Design review of the part built by this model. Coordinates are the model's own, in mm. A direction names the side the tool comes from. Give positions to 0.01 mm unless a question says otherwise; leave off trailing zeros. Order: outer loops, then holes, each group sorted by start corner. A loop starts at its lowest first (then second) coordinate and runs counter-clockwise, first axis right, second up. Notation, with made-up numbers: (-2.5, -9.75) -> (19.5, -9.75) arc R28 ccw to (19.5, 15.25) -> close; hole circle Ø4 at (-9.75, -7.5). An arc over 180 degrees is marked (long way). Answer in a Markdown table with one row per item. Add a question column.
```python
from build123d import *

# Parameters (mm, degrees)
F0_R     = 4.0005
F0_R_2   = 2.9972
F1_DEPTH = 2.032
F2_R     = 2.54
F3_DEPTH = 5.08
F4_R     = 1.9939
F5_DEPTH = 7.2898
F6_R     = 1.781887
F7_DEPTH = 0.254


with BuildPart() as f1:
    # F0 (on Front) → F1 (new body)
    with BuildSketch(Plane.XZ):
        Circle(F0_R)
        Circle(F0_R_2, mode=Mode.SUBTRACT)
        Circle(F0_R_2)
    extrude(amount=F1_DEPTH)

    # F2 (on face) → F3 (join)
    with BuildSketch(Plane(origin=(0, 0, 0), x_dir=(-1, 0, 0), z_dir=(0, 1, 0))):
        Circle(F2_R)
    extrude(amount=F3_DEPTH)

    # F4 (on face) → F5 (join)
    with BuildSketch(Plane(origin=(0, 5.08, 0), x_dir=(-1, 0, 0), z_dir=(0, 1, 0))):
        Circle(F4_R)
    extrude(amount=F5_DEPTH)

    # F6 (on face) → F7 (join)
    with BuildSketch(Plane(origin=(0, 12.3698, 0), x_dir=(-1, 0, 0), z_dir=(0, 1, 0))):
        Circle(F6_R)
    extrude(amount=F7_DEPTH)


solid = f1.part
```
1) Clearance check with flat-ended pins moving along their axes: P1, Ø2, axis at x = 2.5, y = 9, coming from the -Z side; P2, Ø4, axis at y = 2.5, z = -1, coming from the +X side; P3, Ø4, axis at y = 6.5, z = -2.5, coming from the -X side. State where each tip first meets the part, or that it passes through.
2) Machinability: for faces 1 (the face through (-0.9, -1, -3.9)), 2 (the face through (0.33, 2.5, 2.52)), which of the approach directions +Z, -Z, +X, -X, +Y, -Y give a long, thin tool a straight path to every point of the face, cutting with its end or side? Answer none if there is none.
3) Add section A-A, the plane z = 0. Write out the cut boundary in (x, y).
4) For L1, parallel to Y at x = -3.5, z = 0.5; L2, parallel to Z at x = 0, y = 10; L3, parallel to Y at x = 0.5, z = 1.75, list the stretches that pass through material, from the lowest coordinate up.
5) Add section C-C, the plane y = 10. Write out the cut boundary in (x, z), and give its area (3 significant figures).
6) Add section D-D, the plane y = 1.5. Write out the cut boundary in (x, z), and give its area (3 significant figures).
7) Add section B-B, the plane x = 0. Write out the cut boundary in (y, z), and give its area (3 significant figures).
Verdict:
| question | item | result |
|---|---|---|
| 1 | P1 | stops at z = -1.31 |
| 1 | P2 | stops at x = 2.54 |
| 1 | P3 | stops at x = -2.29 |
| 2 | face 1 | +Y, -Y |
| 2 | face 2 | +Y |
| 3 | outline | (-4, -2.03) -> (4, -2.03) -> (4, 0) -> (2.54, 0) -> (2.54, 5.08) -> (1.99, 5.08) -> (1.99, 12.37) -> (1.78, 12.37) -> (1.78, 12.62) -> (-1.78, 12.62) -> (-1.78, 12.37) -> (-1.99, 12.37) -> (-1.99, 5.08) -> (-2.54, 5.08) -> (-2.54, 0) -> (-4, 0) -> close |
| 4 | L1 | y = -2.03 to 0 |
| 4 | L2 | z = -1.99 to 1.99 |
| 4 | L3 | y = -2.03 to 12.37 |
| 5 | outline | circle Ø3.99 at (0, 0) |
| 5 | area | 12.5 mm2 |
| 6 | outline | circle Ø5.08 at (0, 0) |
| 6 | area | 20.3 mm2 |
| 7 | outline | (-2.03, -4) -> (0, -4) -> (0, -2.54) -> (5.08, -2.54) -> (5.08, -1.99) -> (12.37, -1.99) -> (12.37, -1.78) -> (12.62, -1.78) -> (12.62, 1.78) -> (12.37, 1.78) -> (12.37, 1.99) -> (5.08, 1.99) -> (5.08, 2.54) -> (0, 2.54) -> (0, 4) -> (-2.03, 4) -> close |
| 7 | area | 72.0 mm2 |
